Geometry: final body of the model. Coordinates: model frame, mm. Round coordinates to 2 decimals unless told otherwise and drop trailing zeros. Loops run counter-clockwise (first coordinate to the right, second up) from the corner with the lowest first, then second, coordinate; pieces in that order, holes last. Notation, with made-up numbers: M -24,-22 L 33,-22 A31 ccw 33,16 Z; hole C 39.25,50.5 d11. An arc over 180 degrees is marked long. Write each question's results on one line, items separated by ' | '.
```python
from build123d import *

# Parameters (mm, degrees)
SKETCH_1_R          = 1.75
SKETCH_1_R_2        = 1.65
EXTRUDE_1_DEPTH     = 2.2
SKETCH_10_R         = 0.8
SKETCH_10_R_2       = 0.7
EXTRUDE_2_DEPTH     = 1.2
SKETCH_11_R         = 0.8
SKETCH_11_R_2       = 0.7
EXTRUDE_4_DEPTH     = 0.9
SKETCH_12_W         = 0.3
SKETCH_12_H         = 0.9
SKETCH_13_R         = 0.85
CUT_EXTRUDE_2_DEPTH = 0.5
CHAMFER_1_SIZE      = 0.15
CHAMFER_1_SIZE_2    = 0.259807621
SKETCH_14_R         = 1.1
SKETCH_14_R_2       = 0.85
EXTRUDE_5_DEPTH     = 0.6
SKETCH_15_R         = 1.35
SKETCH_15_R_2       = 1.1
EXTRUDE_6_DEPTH     = 0.8
SKETCH_17_R         = 1.1
SKETCH_17_R_2       = 0.85
EXTRUDE_7_DEPTH     = 0.8
CHAMFER_3_SIZE      = 0.2
CUT_EXTRUDE_START   = -0.35
SKETCH_20_R         = 1.35
SKETCH_20_R_2       = 0.85
CUT_EXTRUDE_4_DEPTH = 0.35


with BuildPart() as part:
    # Sketch 1 → Extrude 1 (new body)
    with BuildSketch(Plane.XY):
        Circle(SKETCH_1_R)
        Circle(SKETCH_1_R_2, mode=Mode.SUBTRACT)
    extrude(amount=EXTRUDE_1_DEPTH)

    # Sketch 2 → Revolve 1 (revolve)
    with BuildSketch(Plane(origin=(0, 0, 0), x_dir=(1, 0, 0), z_dir=(0, 1, 0)), mode=Mode.PRIVATE) as revolve_1_sk:
        Polygon((2, -1.6), (1.75, -1.8), (1.75, -1.6), align=None)
    revolve(revolve_1_sk.sketch.rotate(Axis((0, 0, 0), (0, 0, 1)), 180), axis=Axis((0, 0, 0), (0, 0, 1)))

    # Sketch 3 → Revolve 2 (revolve)
    with BuildSketch(Plane(origin=(0, 0, 0), x_dir=(1, 0, 0), z_dir=(0, 1, 0)), mode=Mode.PRIVATE) as revolve_2_sk:
        Polygon((0.8, -3), (1.75, -2.2), (1.65, -2.2), (0.8, -2.915789474), align=None)
    revolve(revolve_2_sk.sketch.rotate(Axis((0, 0, 0), (0, 0, 1)), 180), axis=Axis((0, 0, 0), (0, 0, 1)))

    # Sketch 10 → Extrude 2 (add, symmetric)
    with BuildSketch(Plane(origin=(0, 0, 2.8), x_dir=(-1, 0, 0), z_dir=(0, 0, -1))):
        Circle(SKETCH_10_R)
        Circle(SKETCH_10_R_2, mode=Mode.SUBTRACT)
    extrude(amount=EXTRUDE_2_DEPTH, both=True)

    # Sketch 11 → Extrude 4 (add)
    with BuildSketch(Plane.XY.offset(4)):
        with Locations(Location((0, 0, 0), (0, 0, 180))):
            Circle(SKETCH_11_R)
        Circle(SKETCH_11_R_2, mode=Mode.SUBTRACT)
    extrude(amount=EXTRUDE_4_DEPTH)

    # Sketch 12 → Revolve 3 (revolve)
    with BuildSketch(Plane(origin=(0, 0, 0), x_dir=(1, 0, 0), z_dir=(0, 1, 0)), mode=Mode.PRIVATE) as revolve_3_sk:
        with Locations((0.95, -4.45)):
            Rectangle(SKETCH_12_W, SKETCH_12_H)
    revolve(revolve_3_sk.sketch.rotate(Axis((0, 0, 0), (0, 0, 1)), 180), axis=Axis((0, 0, 0), (0, 0, 1)))

    # Sketch 13 → Cut-Extrude 2 (cut)
    with BuildSketch(Plane.XY.offset(4.9)):
        Circle(SKETCH_13_R)
    extrude(amount=-CUT_EXTRUDE_2_DEPTH, mode=Mode.SUBTRACT)

    # Chamfer 1
    # the kernel refuses this chamfer: 0.259807621, 0.15 mm, written as the material it takes off along each edge
    with BuildSketch(Plane(origin=(0, 0, 4.4), x_dir=(1, 0, 0), z_dir=(0, 1, 0))) as chamfer_1_piece_1_section:
        Polygon((0.7 + CHAMFER_1_SIZE, 0), (0.7, CHAMFER_1_SIZE_2), (0.7, 0), align=None)
    chamfer_1_piece_1 = revolve(axis=Axis((0, 0, 4.4), (0, 0, -1)), mode=Mode.PRIVATE)
    chamfer_1_piece_1 = chamfer_1_piece_1 & Plane(origin=(0, 0, 4.267945413), x_dir=(1, 0, 0), z_dir=(0, 0, 1)) * Cylinder(0.85, 4, mode=Mode.PRIVATE)
    add(chamfer_1_piece_1, mode=Mode.SUBTRACT)

    # Sketch 14 → Extrude 5 (add)
    with BuildSketch(Plane.XY.offset(4.9)):
        with Locations(Location((0, 0, 0), (0, 0, 180))):
            Circle(SKETCH_14_R)
        Circle(SKETCH_14_R_2, mode=Mode.SUBTRACT)
    extrude(amount=EXTRUDE_5_DEPTH)



with BuildPart() as body_2:
    # Sketch 15 → Extrude 6 (new body)
    with BuildSketch(Plane.XY.offset(5.5)):
        Circle(SKETCH_15_R)
        with Locations(Location((0, 0, 0), (0, 0, 180))):
            Circle(SKETCH_15_R_2, mode=Mode.SUBTRACT)
    extrude(amount=EXTRUDE_6_DEPTH)


with BuildPart() as part_1:
    add(part.part)

    add(body_2.part)  # Extrude 7 merges body 2
    # Sketch 17 → Extrude 7 (add)
    with BuildSketch(Plane.XY.offset(5.5)):
        with Locations(Location((0, 0, 0), (0, 0, 180))):
            Circle(SKETCH_17_R)
        Circle(SKETCH_17_R_2, mode=Mode.SUBTRACT)
    extrude(amount=EXTRUDE_7_DEPTH)

    # Chamfer 3
    chamfer_3_edges = [part_1.edges().sort_by_distance(p)[0] for p in [
        (-1.35, 0, 5.5),
    ]]
    chamfer(chamfer_3_edges, length=CHAMFER_3_SIZE)

    # Sketch 20 → Cut-Extrude 4 (cut)
    with BuildSketch(Plane.XY.offset(6.3).offset(CUT_EXTRUDE_START)):
        Circle(SKETCH_20_R)
        Circle(SKETCH_20_R_2, mode=Mode.SUBTRACT)
        with BuildLine():
            Line((-0.940452019, -0.940452019), (0.076720819, -0.876922974))
            ThreePointArc((0.076720819, -0.876922974), (-0.414209233, -1.191386171), (-0.940452019, -0.940452019))
        make_face(mode=Mode.SUBTRACT)
        with BuildLine():
            Line((-1.33, 0), (-0.56582837, -0.674327993))
            ThreePointArc((-0.56582837, -0.674327993), (-1.135327398, -0.549547083), (-1.33, 0))
        make_face(mode=Mode.SUBTRACT)
        with BuildLine():
            Line((0, -1.33), (0.674327993, -0.56582837))
            ThreePointArc((0.674327993, -0.56582837), (0.549547083, -1.135327398), (0, -1.33))
        make_face(mode=Mode.SUBTRACT)
        with BuildLine():
            Line((0.940452019, -0.940452019), (0.876922974, 0.076720819))
            ThreePointArc((0.876922974, 0.076720819), (1.191386171, -0.414209233), (0.940452019, -0.940452019))
        make_face(mode=Mode.SUBTRACT)
        with BuildLine():
            Line((-0.940452019, 0.940452019), (-0.876922974, -0.076720819))
            ThreePointArc((-0.876922974, -0.076720819), (-1.191386171, 0.414209233), (-0.940452019, 0.940452019))
        make_face(mode=Mode.SUBTRACT)
        with BuildLine():
            ThreePointArc((-0.674327993, 0.56582837), (-0.549547083, 1.135327398), (0, 1.33))
            Line((0, 1.33), (-0.674327993, 0.56582837))
        make_face(mode=Mode.SUBTRACT)
        with BuildLine():
            Line((0.940452019, 0.940452019), (-0.076720819, 0.876922974))
            ThreePointArc((-0.076720819, 0.876922974), (0.414209233, 1.191386171), (0.940452019, 0.940452019))
        make_face(mode=Mode.SUBTRACT)
        with BuildLine():
            Line((1.33, 0), (0.56582837, 0.674327993))
            ThreePointArc((0.56582837, 0.674327993), (1.135327398, 0.549547083), (1.33, 0))
        make_face(mode=Mode.SUBTRACT)
    extrude(amount=CUT_EXTRUDE_4_DEPTH, mode=Mode.SUBTRACT)


solid = part_1.part
```
1. Section B-B (z = 5.25). Output: boundary loops of the cut face in (x, y).
Answer key:
outline: C 0,0 d2.2; hole C 0,0 d1.7
2. Section A-A (z = 1.25). Output: boundary loops of the cut face in (x, y).
Answer key:
outline: C 0,0 d3.5; hole C 0,0 d3.3
3. Ray query, probe 1 along Y at (x, z) = (0.75, 6.25); probe 2 along X at (y, z) = (-0.25, 4.75); probe 3 along X at (y, z) = (-0.25, 5.75). Return the intervals inside material, ascending.
Answer key:
probe 1: y = 0.51 to 0.7, 0.93 to 1.11 | probe 2: x = -1.07 to -0.81, 0.81 to 1.07 | probe 3: x = -1.33 to -0.81, 0.81 to 1.33
4. Pin query (flat end, axial travel): P1, Ø1.6, axis at x = 0, y = 0, coming from the +Z side; P2, Ø2, axis at y = 1, z = 0.5, coming from the +X side; P3, Ø0.5, axis at x = 0, y = 0.5, coming from the -Z side. Return the tip coordinate at first contact, or that it passes through.
Answer key:
P1: stops at z = 4.31 | P2: stops at x = 1.75 | P3: stops at z = 1.6
